from build123d import *

# Parameters (mm, degrees)
BOSS_EXTRUDE1_DEPTH                            = 10
CBORE_START                                    = -1
CBORE_SLOT_FOR_M3_HEX_HEAD_MACHINE_SCREW_DEPTH = 4.3
CBORE_START_2                                  = 3.3
CBORE_SLOT_FOR_M3_HEX_HEAD_MACHINE_S_3_DEPTH   = 7.7
SKETCH12_R                                     = 1.25
CUT_EXTRUDE4_DEPTH                             = 114.578166925
SKETCH12_5_R                                   = 5.1
CUT_EXTRUDE5_DEPTH                             = 8.85
SKETCH12_6_W                                   = 45.4
SKETCH12_6_H                                   = 24.5
CUT_EXTRUDE6_DEPTH                             = 2.9
SKETCH16_R                                     = 2
CUT_EXTRUDE7_DEPTH                             = 2.5


with BuildPart() as part:
    # Sketch1 → Boss-Extrude1 (new body)
    with BuildSketch(Plane.XY):
        with BuildLine():
            Line((-59.529404499, 7.5), (-75, 7.5))
            Line((-75, 7.5), (-80, 2.5))
            Line((-80, 2.5), (-80, -2.5))
            Line((-80, -2.5), (-75, -7.5))
            Line((-75, -7.5), (-59.529404499, -7.5))
            ThreePointArc((-59.529404499, -7.5), (-42.426406871, -42.426406871), (-7.5, -59.529404499))
            Line((-7.5, -59.529404499), (-7.5, -75))
            Line((-7.5, -75), (-2.5, -80))
            Line((-2.5, -80), (2.5, -80))
            Line((2.5, -80), (7.5, -75))
            Line((7.5, -75), (7.5, -59.529404499))
            ThreePointArc((7.5, -59.529404499), (42.426406871, -42.426406871), (59.529404499, -7.5))
            Line((59.529404499, -7.5), (75, -7.5))
            Line((75, -7.5), (80, -2.5))
            Line((80, -2.5), (80, 2.5))
            Line((80, 2.5), (75, 7.5))
            Line((75, 7.5), (59.529404499, 7.5))
            ThreePointArc((59.529404499, 7.5), (42.426406871, 42.426406871), (7.5, 59.529404499))
            Line((7.5, 59.529404499), (7.5, 75))
            Line((7.5, 75), (2.5, 80))
            Line((2.5, 80), (-2.5, 80))
            Line((-2.5, 80), (-7.5, 75))
            Line((-7.5, 75), (-7.5, 59.529404499))
            ThreePointArc((-7.5, 59.529404499), (-42.426406871, 42.426406871), (-59.529404499, 7.5))
        make_face()
    extrude(amount=BOSS_EXTRUDE1_DEPTH)

    # CBORE SLOT for M3 Hex Head Machine Screw1: read off the stored shape, not the designer's step
    # CBORE SLOT for M3 Hex Head Machine S 2 → CBORE SLOT for M3 Hex Head Machine Screw1 (cut)
    with BuildSketch(Plane.XY.offset(CBORE_START)):
        with BuildLine():
            ThreePointArc((0.05, 65.8), (4.25, 70), (0.05, 74.2))
            Line((0.05, 74.2), (-0.05, 74.2))
            ThreePointArc((-0.05, 74.2), (-4.25, 70), (-0.05, 65.8))
            Line((-0.05, 65.8), (0.05, 65.8))
        make_face()
        with BuildLine():
            ThreePointArc((-69.95, -4.2), (-65.75, 0), (-69.95, 4.2))
            Line((-69.95, 4.2), (-70.05, 4.2))
            ThreePointArc((-70.05, 4.2), (-74.25, 0), (-70.05, -4.2))
            Line((-70.05, -4.2), (-69.95, -4.2))
        make_face()
        with BuildLine():
            ThreePointArc((69.95, 4.2), (65.75, 0), (69.95, -4.2))
            Line((69.95, -4.2), (70.05, -4.2))
            ThreePointArc((70.05, -4.2), (74.25, 0), (70.05, 4.2))
            Line((70.05, 4.2), (69.95, 4.2))
        make_face()
        with BuildLine():
            ThreePointArc((0.05, -74.2), (4.25, -70), (0.05, -65.8))
            Line((0.05, -65.8), (-0.05, -65.8))
            ThreePointArc((-0.05, -65.8), (-4.25, -70), (-0.05, -74.2))
            Line((-0.05, -74.2), (0.05, -74.2))
        make_face()
    extrude(amount=CBORE_SLOT_FOR_M3_HEX_HEAD_MACHINE_SCREW_DEPTH, mode=Mode.SUBTRACT)

    # CBORE SLOT for M3 Hex Head Machine S 3 o → CBORE SLOT for M3 Hex Head Machine S 3 (cut)
    with BuildSketch(Plane.XY.offset(CBORE_START_2)):
        with BuildLine():
            ThreePointArc((0.05, 68.3), (1.75, 70), (0.05, 71.7))
            Line((0.05, 71.7), (-0.05, 71.7))
            ThreePointArc((-0.05, 71.7), (-1.75, 70), (-0.05, 68.3))
            Line((-0.05, 68.3), (0.05, 68.3))
        make_face()
        with BuildLine():
            ThreePointArc((-69.95, -1.7), (-68.25, 0), (-69.95, 1.7))
            Line((-69.95, 1.7), (-70.05, 1.7))
            ThreePointArc((-70.05, 1.7), (-71.75, 0), (-70.05, -1.7))
            Line((-70.05, -1.7), (-69.95, -1.7))
        make_face()
        with BuildLine():
            ThreePointArc((69.95, 1.7), (68.25, 0), (69.95, -1.7))
            Line((69.95, -1.7), (70.05, -1.7))
            ThreePointArc((70.05, -1.7), (71.75, 0), (70.05, 1.7))
            Line((70.05, 1.7), (69.95, 1.7))
        make_face()
        with BuildLine():
            ThreePointArc((0.05, -71.7), (1.75, -70), (0.05, -68.3))
            Line((0.05, -68.3), (-0.05, -68.3))
            ThreePointArc((-0.05, -68.3), (-1.75, -70), (-0.05, -71.7))
            Line((-0.05, -71.7), (0.05, -71.7))
        make_face()
    extrude(amount=CBORE_SLOT_FOR_M3_HEX_HEAD_MACHINE_S_3_DEPTH, mode=Mode.SUBTRACT)

    # CBORE SLOT for M3 Hex Head Machine S 4: loft between two sections, ruled curve by curve
    cbore_slot_for_m3_hex_head_machine_s_4_from = [
        Edge.make_three_point_arc((0.05, 74.2, 0.025), (3.019848481, 72.969848481, 0.025), (4.25, 70, 0.025)),
        Edge.make_three_point_arc((4.25, 70, 0.025), (3.019848481, 67.030151519, 0.025), (0.05, 65.8, 0.025)),
        Edge.make_three_point_arc((-0.05, 65.8, 0.025), (-3.019848481, 67.030151519, 0.025), (-4.25, 70, 0.025)),
        Edge.make_three_point_arc((-4.25, 70, 0.025), (-3.019848481, 72.969848481, 0.025), (-0.05, 74.2, 0.025)),
        Edge.make_line((0.05, 65.8, 0.025), (-0.05, 65.8, 0.025)),
        Edge.make_line((0.05, 74.2, 0.025), (-0.05, 74.2, 0.025)),
    ]
    cbore_slot_for_m3_hex_head_machine_s_4_to = [
        Edge.make_three_point_arc((0.05, 74.225, 0), (3.037526151, 72.987526151, 0), (4.275, 70, 0)),
        Edge.make_three_point_arc((4.275, 70, 0), (3.037526151, 67.012473849, 0), (0.05, 65.775, 0)),
        Edge.make_three_point_arc((-0.05, 65.775, 0), (-3.037526151, 67.012473849, 0), (-4.275, 70, 0)),
        Edge.make_three_point_arc((-4.275, 70, 0), (-3.037526151, 72.987526151, 0), (-0.05, 74.225, 0)),
        Edge.make_line((0.05, 65.775, 0), (-0.05, 65.775, 0)),
        Edge.make_line((0.05, 74.225, 0), (-0.05, 74.225, 0)),
    ]
    cbore_slot_for_m3_hex_head_machine_s_4 = Solid(Shell([*[Face.make_surface_from_curves(cbore_slot_for_m3_hex_head_machine_s_4_from[k], cbore_slot_for_m3_hex_head_machine_s_4_to[k]) for k in range(6)], Face(Wire(cbore_slot_for_m3_hex_head_machine_s_4_from)), Face(Wire(cbore_slot_for_m3_hex_head_machine_s_4_to))]))
    add(cbore_slot_for_m3_hex_head_machine_s_4, mode=Mode.SUBTRACT)

    # CBORE SLOT for M3 Hex Head Machine S 5: loft between two sections, ruled curve by curve
    cbore_slot_for_m3_hex_head_machine_s_5_from = [
        Edge.make_three_point_arc((-69.95, 4.2, 0.025), (-66.980151519, 2.969848481, 0.025), (-65.75, 0, 0.025)),
        Edge.make_three_point_arc((-65.75, 0, 0.025), (-66.980151519, -2.969848481, 0.025), (-69.95, -4.2, 0.025)),
        Edge.make_three_point_arc((-70.05, -4.2, 0.025), (-73.019848481, -2.969848481, 0.025), (-74.25, 0, 0.025)),
        Edge.make_three_point_arc((-74.25, 0, 0.025), (-73.019848481, 2.969848481, 0.025), (-70.05, 4.2, 0.025)),
        Edge.make_line((-69.95, -4.2, 0.025), (-70.05, -4.2, 0.025)),
        Edge.make_line((-69.95, 4.2, 0.025), (-70.05, 4.2, 0.025)),
    ]
    cbore_slot_for_m3_hex_head_machine_s_5_to = [
        Edge.make_three_point_arc((-69.95, 4.225, 0), (-66.962473849, 2.987526151, 0), (-65.725, 0, 0)),
        Edge.make_three_point_arc((-65.725, 0, 0), (-66.962473849, -2.987526151, 0), (-69.95, -4.225, 0)),
        Edge.make_three_point_arc((-70.05, -4.225, 0), (-73.037526151, -2.987526151, 0), (-74.275, 0, 0)),
        Edge.make_three_point_arc((-74.275, 0, 0), (-73.037526151, 2.987526151, 0), (-70.05, 4.225, 0)),
        Edge.make_line((-69.95, -4.225, 0), (-70.05, -4.225, 0)),
        Edge.make_line((-69.95, 4.225, 0), (-70.05, 4.225, 0)),
    ]
    cbore_slot_for_m3_hex_head_machine_s_5 = Solid(Shell([*[Face.make_surface_from_curves(cbore_slot_for_m3_hex_head_machine_s_5_from[k], cbore_slot_for_m3_hex_head_machine_s_5_to[k]) for k in range(6)], Face(Wire(cbore_slot_for_m3_hex_head_machine_s_5_from)), Face(Wire(cbore_slot_for_m3_hex_head_machine_s_5_to))]))
    add(cbore_slot_for_m3_hex_head_machine_s_5, mode=Mode.SUBTRACT)

    # CBORE SLOT for M3 Hex Head Machine S 6: loft between two sections, ruled curve by curve
    cbore_slot_for_m3_hex_head_machine_s_6_from = [
        Edge.make_three_point_arc((70.05, 4.2, 0.025), (73.019848481, 2.969848481, 0.025), (74.25, 0, 0.025)),
        Edge.make_three_point_arc((74.25, 0, 0.025), (73.019848481, -2.969848481, 0.025), (70.05, -4.2, 0.025)),
        Edge.make_three_point_arc((69.95, -4.2, 0.025), (66.980151519, -2.969848481, 0.025), (65.75, 0, 0.025)),
        Edge.make_three_point_arc((65.75, 0, 0.025), (66.980151519, 2.969848481, 0.025), (69.95, 4.2, 0.025)),
        Edge.make_line((70.05, -4.2, 0.025), (69.95, -4.2, 0.025)),
        Edge.make_line((70.05, 4.2, 0.025), (69.95, 4.2, 0.025)),
    ]
    cbore_slot_for_m3_hex_head_machine_s_6_to = [
        Edge.make_three_point_arc((70.05, 4.225, 0), (73.037526151, 2.987526151, 0), (74.275, 0, 0)),
        Edge.make_three_point_arc((74.275, 0, 0), (73.037526151, -2.987526151, 0), (70.05, -4.225, 0)),
        Edge.make_three_point_arc((69.95, -4.225, 0), (66.962473849, -2.987526151, 0), (65.725, 0, 0)),
        Edge.make_three_point_arc((65.725, 0, 0), (66.962473849, 2.987526151, 0), (69.95, 4.225, 0)),
        Edge.make_line((70.05, -4.225, 0), (69.95, -4.225, 0)),
        Edge.make_line((70.05, 4.225, 0), (69.95, 4.225, 0)),
    ]
    cbore_slot_for_m3_hex_head_machine_s_6 = Solid(Shell([*[Face.make_surface_from_curves(cbore_slot_for_m3_hex_head_machine_s_6_from[k], cbore_slot_for_m3_hex_head_machine_s_6_to[k]) for k in range(6)], Face(Wire(cbore_slot_for_m3_hex_head_machine_s_6_from)), Face(Wire(cbore_slot_for_m3_hex_head_machine_s_6_to))]))
    add(cbore_slot_for_m3_hex_head_machine_s_6, mode=Mode.SUBTRACT)

    # CBORE SLOT for M3 Hex Head Machine S 7: loft between two sections, ruled curve by curve
    cbore_slot_for_m3_hex_head_machine_s_7_from = [
        Edge.make_three_point_arc((0.05, -65.8, 0.025), (3.019848481, -67.030151519, 0.025), (4.25, -70, 0.025)),
        Edge.make_three_point_arc((4.25, -70, 0.025), (3.019848481, -72.969848481, 0.025), (0.05, -74.2, 0.025)),
        Edge.make_three_point_arc((-0.05, -74.2, 0.025), (-3.019848481, -72.969848481, 0.025), (-4.25, -70, 0.025)),
        Edge.make_three_point_arc((-4.25, -70, 0.025), (-3.019848481, -67.030151519, 0.025), (-0.05, -65.8, 0.025)),
        Edge.make_line((0.05, -74.2, 0.025), (-0.05, -74.2, 0.025)),
        Edge.make_line((0.05, -65.8, 0.025), (-0.05, -65.8, 0.025)),
    ]
    cbore_slot_for_m3_hex_head_machine_s_7_to = [
        Edge.make_three_point_arc((0.05, -65.775, 0), (3.037526151, -67.012473849, 0), (4.275, -70, 0)),
        Edge.make_three_point_arc((4.275, -70, 0), (3.037526151, -72.987526151, 0), (0.05, -74.225, 0)),
        Edge.make_three_point_arc((-0.05, -74.225, 0), (-3.037526151, -72.987526151, 0), (-4.275, -70, 0)),
        Edge.make_three_point_arc((-4.275, -70, 0), (-3.037526151, -67.012473849, 0), (-0.05, -65.775, 0)),
        Edge.make_line((0.05, -74.225, 0), (-0.05, -74.225, 0)),
        Edge.make_line((0.05, -65.775, 0), (-0.05, -65.775, 0)),
    ]
    cbore_slot_for_m3_hex_head_machine_s_7 = Solid(Shell([*[Face.make_surface_from_curves(cbore_slot_for_m3_hex_head_machine_s_7_from[k], cbore_slot_for_m3_hex_head_machine_s_7_to[k]) for k in range(6)], Face(Wire(cbore_slot_for_m3_hex_head_machine_s_7_from)), Face(Wire(cbore_slot_for_m3_hex_head_machine_s_7_to))]))
    add(cbore_slot_for_m3_hex_head_machine_s_7, mode=Mode.SUBTRACT)

    # Sketch12 → Cut-Extrude4 (cut, through all)
    with BuildSketch(Plane.XY.offset(10)):
        with Locations((4.85, 15)):
            Circle(SKETCH12_R)
        with Locations((-12.15, 15)):
            Circle(SKETCH12_R)
        with Locations((-29.15, 15)):
            Circle(SKETCH12_R)
        with Locations(Location((-29.15, -15, 0), (0, 0, 180))):
            Circle(SKETCH12_R)
        with Locations(Location((-12.15, -15, 0), (0, 0, 180))):
            Circle(SKETCH12_R)
        with Locations(Location((4.85, -15, 0), (0, 0, 180))):
            Circle(SKETCH12_R)
    extrude(amount=-CUT_EXTRUDE4_DEPTH, mode=Mode.SUBTRACT)

    # Sketch12<5> → Cut-Extrude5 (cut)
    with BuildSketch(Plane.XY.offset(10)):
        Circle(SKETCH12_5_R)
    extrude(amount=-CUT_EXTRUDE5_DEPTH, mode=Mode.SUBTRACT)

    # Sketch12<6> → Cut-Extrude6 (cut)
    with BuildSketch(Plane.XY.offset(10)):
        with Locations((-10.35, 0)):
            Rectangle(SKETCH12_6_W, SKETCH12_6_H)
    extrude(amount=-CUT_EXTRUDE6_DEPTH, mode=Mode.SUBTRACT)

    # Sketch16 → Cut-Extrude7 (cut)
    with BuildSketch(Plane(origin=(0, 0, 0), x_dir=(-1, 0, 0), z_dir=(0, 0, -1))):
        with Locations((-4.85, 15)):
            Circle(SKETCH16_R)
        with Locations((12.15, 15)):
            Circle(SKETCH16_R)
        with Locations((29.15, 15)):
            Circle(SKETCH16_R)
        with Locations((-4.85, -15)):
            Circle(SKETCH16_R)
        with Locations((12.15, -15)):
            Circle(SKETCH16_R)
        with Locations((29.15, -15)):
            Circle(SKETCH16_R)
    extrude(amount=-CUT_EXTRUDE7_DEPTH, mode=Mode.SUBTRACT)


solid = part.part
Can you work these out from the model? Positions are in its coordinate system, mm. A direction names the side the tool comes from. Give positions to 0.01 mm unless a question says otherwise; leave off trailing zeros. Loops run counter-clockwise (first coordinate to the right, second up) from the corner with the lowest first, then second, coordinate; pieces in that order, holes last. Notation, with made-up numbers: (15, 75) - (65, 75) arc R7 ccw to (65, 84) - close; hole circle Ø8 at (56, -13). An arc over 180 degrees is marked (long way). Return JSON: item names as keys, results as strings.
1. For faces 1 (the face through (7.5, -67, 5)), 2 (the face through (1.75, -70.04, 6.6)), 3 (the face through (-28, -16, 2.5)), which set-ups out of +Z, -Z, +X, -X, +Y, -Y let a thin tool reach every point of the face, with its end or its side?
Output values:
{"face 1": "+Z, -Z, +X, -Y", "face 2": "+Z, -Z", "face 3": "-Z"}
2. I'm going to push flat-ended pins straight in: pin 1 Ø3 at (y, z) = (48.5, 3) entering from +X; pin 2 Ø1.2 at (x, y) = (4.5, -15) entering from -Z (3 decimals); pin 3 Ø6 at (x, z) = (29, 7.5) entering from +Y; pin 4 Ø3 at (y, z) = (64.5, 7.5) entering from +X. Where does each tip first touch, or does it pass through?
Output values:
{"pin 1": "stops at x = 37.3", "pin 2": "passes through", "pin 3": "stops at y = 54.07", "pin 4": "stops at x = 7.5"}
3. I want a section at A-A on z = 5. Give the number of separate pieces and of enclosed holes in the cut face, and give its area (3 significant figures).
Output values:
{"separate pieces": "1", "enclosed holes": "11", "area": "12,300 mm²"}
4. We'd pull the mould along X, two halves only. Please class faces 4 (the face through (5, 77.5, 4.9)), 5 (the face through (-5, -77.5, 4.9)), 6 (the face through (-13.2, 16.7, 1.2)): +X half, -X half, draft (parallel to the pull), parting line (faces both ways), or undercut.
Output values:
{"face 4": "+X half", "face 5": "-X half", "face 6": "undercut"}
5. I want a section at C-C on y = 38. Please give me the cut outline in (x, z).
Output values:
{"outline": "(-46.43, 0) - (46.43, 0) - (46.43, 10) - (-46.43, 10) - close"}
6. I want a section at B-B on x = -52. Please give me the cut outline in (y, z), and give its area (3 significant figures).
Output values:
{"outline": "(-29.93, 0) - (29.93, 0) - (29.93, 10) - (-29.93, 10) - close", "area": "599 mm²"}
7. If I drill on line 1 (Y direction, x = 0, z = 7.5); line 2 (Y direction, x = -12.15, z = 0.5); line 3 (Y direction, x = -29.5, z = 6), over which ranges is the centre line in solid material (lowest first)?
Output values:
{"line 1": "y = -80 to -71.7, -68.3 to -12.25, 12.25 to 68.3, 71.7 to 80", "line 2": "y = -58.76 to -17, -13 to 13, 17 to 58.76", "line 3": "y = -52.25 to -16.2, -13.8 to 13.8, 16.2 to 52.25"}
